The drawing under review shows one solid part. Ordinate dimensions are in mm from its lowest x, y, z. A direction names the side the tool comes from. Round coordinates to 2 decimals unless told otherwise and drop trailing zeros. Order: outer loops, then holes, each group sorted by start corner. A loop starts at its lowest first (then second) coordinate and runs counter-clockwise, first axis right, second up. Notation, with made-up numbers: (48.5, 58) -> (87.5, 58) arc R27 ccw to (87.5, 82) -> close; hole circle Ø3 at (84, -23). An arc over 180 degrees is marked (long way). Use a Markdown table: item, result. Add a question column.
1) Consider section A-A (y = 16.5). State the section outline as (x, z) points.
2) Consider section B-B (x = 28). State the section outline as (y, z) points.
3) Consider section C-C (z = 129). State the section outline as (x, y) points, plus the area to 3 significant figures.
4) Wall thickness on line 1 along X through (y, z) = (3.95, 23); line 2 along Z through (x, y) = (27.5, 12); line 3 along X through (y, z) = (19, 116): over which ranges is each line inside the solid? List them lowest first. Write a range as [from, to].
5) Machinability: for the marked faces 1 and 2, which of the approach directions +Z, -Z, +X, -X, +Y, -Y give a long, thin tool a straight path to every point of the face, cutting with its end or side? Answer none if there is none.
6) Clearance check with flat-ended pins moving along their axes: P1, Ø1.5, axis at y = 2, z = 93, coming from the -X side; P2, Ø6, axis at y = 58.5, z = 22, coming from the -X side; P3, Ø4, axis at x = 25, y = 3.5, coming from the +Z side. State where each tip first meets the part, or that it passes through.
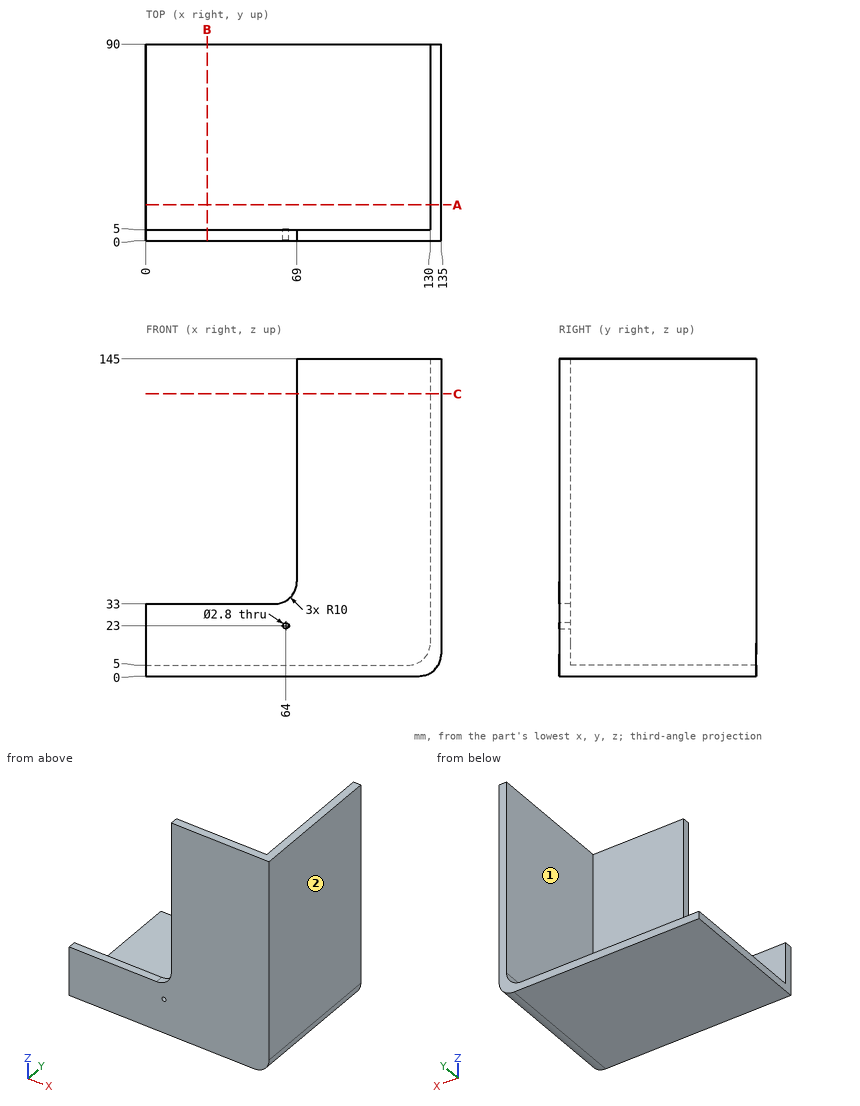
Results list:
| question | item | result |
|---|---|---|
| 1 | outline | (0, 0) -> (125, 0) arc R10 ccw to (135, 10) -> (135, 145) -> (130, 145) -> (130, 15) arc R10 cw to (120, 5) -> (0, 5) -> close |
| 2 | outline | (0, 0) -> (90, 0) -> (90, 5) -> (5, 5) -> (5, 33) -> (0, 33) -> close |
| 3 | outline | (69, 0) -> (135, 0) -> (135, 90) -> (130, 90) -> (130, 5) -> (69, 5) -> close |
| 3 | area | 755 mm2 |
| 4 | line 1 | [0, 62.6], [65.4, 135] |
| 4 | line 2 | [0, 5] |
| 4 | line 3 | [130, 135] |
| 5 | face 1 | +Z, -X, +Y |
| 5 | face 2 | +Z, -Z, +X, +Y, -Y |
| 6 | P1 | x = 69 |
| 6 | P2 | x = 130 |
| 6 | P3 | z = 33 |
